from build123d import *

# Parameters (mm, degrees)
SKETCH1_R           = 6
BOSS_EXTRUDE1_DEPTH = 12
BOSS_EXTRUDE2_START = -25
SKETCH2_W           = 144
SKETCH2_H           = 12
BOSS_EXTRUDE2_DEPTH = 50


with BuildPart() as part:
    # Sketch1 → Boss-Extrude1 (new body)
    with BuildSketch(Plane.XY):
        with BuildLine():
            Line((-72, 0), (72, 0))
            Line((72, 0), (72, 12))
            ThreePointArc((72, 12), (46.579087682, 25.10523588), (32.5, 50))
            Line((32.5, 50), (-32.5, 50))
            ThreePointArc((-32.5, 50), (-46.579087682, 25.10523588), (-72, 12))
            Line((-72, 12), (-72, 0))
        make_face()
        with Locations((19, 31)):
            Circle(SKETCH1_R, mode=Mode.SUBTRACT)
        with Locations(Location((-19, 31, 0), (0, 0, 180))):
            Circle(SKETCH1_R, mode=Mode.SUBTRACT)
    extrude(amount=BOSS_EXTRUDE1_DEPTH)


with BuildPart() as body_2:
    # Mirror2: mirrored copy
    add(part.part.mirror(Plane.XY.offset(37)))


with BuildPart() as part_1:
    add(part.part)

    add(body_2.part)  # Boss-Extrude2 merges body 2
    # Sketch2 → Boss-Extrude2 (add)
    with BuildSketch(Plane.XY.offset(37).offset(BOSS_EXTRUDE2_START)):
        with Locations((0, 6)):
            Rectangle(SKETCH2_W, SKETCH2_H)
    extrude(amount=BOSS_EXTRUDE2_DEPTH)


solid = part_1.part
Read the model definition and answer for the solid it produces. Units are mm, in the model's axes. A direction names the side the tool comes from. Round coordinates to 2 decimals unless told otherwise and drop trailing zeros. Loops run counter-clockwise (first coordinate to the right, second up) from the corner with the lowest first, then second, coordinate; pieces in that order, holes last. Notation, with made-up numbers: (87, -3.5) - (100, -3.5) arc R30 ccw to (100, 25.5) - close; hole circle Ø11 at (-10.75, 40.5). An arc over 180 degrees is marked (long way). One line per question, with ' | ' between items. Start each with the question number.
Q1. Section D-D on y = 20.5 is taken. Give the vertices of the cut face in (x, z).
Q2. A flat-ended cylindrical pin translates along its axis: pin 1 (10 mm diameter, centred on x = -26.5, z = 21.5, fed in from +Y). Find the tip coordinate at first contact, or state that the pin passes through.
Q3. For a pull along Y with two mould halves and no side action, classify faces 1 (the cylindrical face through (-21.769, 36.323, 68.084)), 2 (the flat face through (-1, 27, 62)), 3 (the cylindrical face through (46.9, 24.8, 5.9)) as +Y half, -Y half, draft (parallel to the pull), parting line (faces both ways), or undercut.
Q4. Section A-A on x = 19 is taken. Give the vertices of the cut face in (y, z).
Q5. For faces 4 (the flat face through (-1, 27, 12)), 5 (the flat face through (-72, 6, 36)), determine the directions among +Z, -Z, +X, -X, +Y, -Y from which every point of the face is accessible in a straight line to the end or side of a thin tool.
Q6. Find the intervals of material crossed by L1, parallel to Y at x = -19, z = 70; L2, parallel to Z at x = 37.5, y = 13; L3, parallel to Y at x = -61, z = 19, in increasing order.
Q7. Section C-C on z = 5.5 is taken. Give the vertices of the cut face in (x, y).
Q8. Section B-B on y = 31 is taken. Give the vertices of the cut face in (x, z).
Established:
1) outline: (-52.11, 0) - (52.11, 0) - (52.11, 12) - (-52.11, 12) - close; (-52.11, 62) - (52.11, 62) - (52.11, 74) - (-52.11, 74) - close
2) pin 1: y = 12
3) face 1: undercut | face 2: draft | face 3: +Y half
4) outline: (0, 0) - (25, 0) - (25, 12) - (12, 12) - (12, 62) - (25, 62) - (25, 74) - (0, 74) - close; (37, 0) - (50, 0) - (50, 12) - (37, 12) - close; (37, 62) - (50, 62) - (50, 74) - (37, 74) - close
5) face 4: +X, -X, +Y | face 5: +Z, -Z, -X, +Y, -Y
6) L1: 0 to 25, 37 to 50 | L2: 0 to 12, 62 to 74 | L3: 0 to 12
7) outline: (-72, 0) - (72, 0) - (72, 12) arc R50 cw to (32.5, 50) - (-32.5, 50) arc R50 cw to (-72, 12) - close; hole circle Ø12 at (-19, 31); hole circle Ø12 at (19, 31)
8) outline: (-41.35, 0) - (-25, 0) - (-25, 12) - (-41.35, 12) - close; (-41.35, 62) - (-25, 62) - (-25, 74) - (-41.35, 74) - close; (-13, 0) - (13, 0) - (13, 12) - (-13, 12) - close; (-13, 62) - (13, 62) - (13, 74) - (-13, 74) - close; (25, 0) - (41.35, 0) - (41.35, 12) - (25, 12) - close; (25, 62) - (41.35, 62) - (41.35, 74) - (25, 74) - close
